Model file for the job. Use its own axes, mm. Round coordinates to 2 decimals unless told otherwise and drop trailing zeros. Write each loop counter-clockwise with the first axis right and the second up, starting at its lowest first coordinate (ties: lowest second). Pieces come first, ordered by that corner, then holes. Notation, with made-up numbers: (15.5, -5) - (23.5, -5) arc R28 ccw to (23.5, 23) - close; hole circle Ø8 at (76.5, 36). An arc over 180 degrees is marked (long way). Answer as a JSON object with one key per item and string values. Group by question number.
from build123d import *

# Parameters (mm, degrees)
SKETCH1_W           = 70
SKETCH1_H           = 200
BOSS_EXTRUDE1_DEPTH = 15
SKETCH1_3_R         = 7.5
CUT_EXTRUDE1_DEPTH  = 5
FILLET1_R           = 15


with BuildPart() as part:
    # Sketch1 → Boss-Extrude1 (new body)
    with BuildSketch(Plane(origin=(0, 0, 0), x_dir=(0, 0, -1), z_dir=(1, 0, 0))):
        Rectangle(SKETCH1_W, SKETCH1_H)
    extrude(amount=BOSS_EXTRUDE1_DEPTH)

    # Sketch1<3> → Cut-Extrude1 (cut)
    with BuildSketch(Plane(origin=(0, 0, 0), x_dir=(0, 0, -1), z_dir=(1, 0, 0))):
        with Locations((0, 80)):
            Circle(SKETCH1_3_R)
        with Locations((0, -80)):
            Circle(SKETCH1_3_R)
    extrude(amount=CUT_EXTRUDE1_DEPTH, mode=Mode.SUBTRACT)

    # Fillet1
    fillet1_edges = [part.edges().sort_by_distance(p)[0] for p in [
        (7.5, -100, -35),
        (7.5, -100, 35),
        (7.5, 100, 35),
        (7.5, 100, -35),
    ]]
    fillet(fillet1_edges, radius=FILLET1_R)


solid = part.part
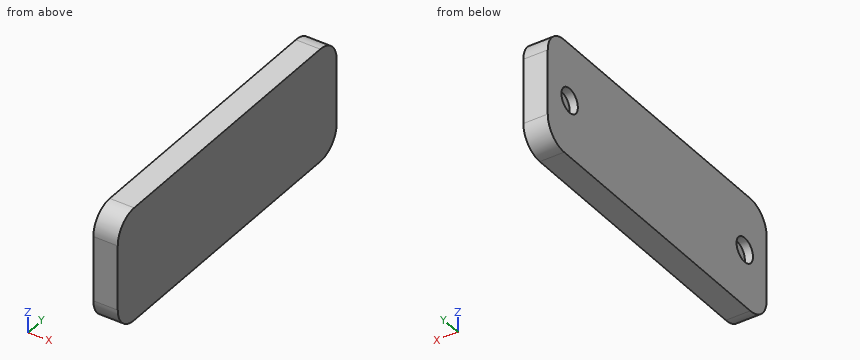
(1) Drill centre lines: line 1 (Y direction, x = 3, z = 0); line 2 (Y direction, x = 9, z = -28); line 3 (Y direction, x = 2.75, z = 26). Where is each one in solid material? Low to high. Write a range as from..to.
(2) Slice it at B-B (z = 0). Write the cut outline in (x, y).
(3) Flat gauge pin, fed straight in: pin 1 (9 mm diameter, centred on y = -80, z = 0, fed in from -X). Where does the tip first touch, or does it go through?
(4) Slice it at A-A (y = -80). Write the cut outline in (x, z), then the cut area to 3 significant figures.
Answer:
{
 "1": {"line 1": "-100..-87.5, -72.5..72.5, 87.5..100", "line 2": "-97.69..97.69", "line 3": "-98.75..98.75"},
 "2": {"outline": "(0, -100) - (15, -100) - (15, 100) - (0, 100) - (0, 87.5) - (5, 87.5) - (5, 72.5) - (0, 72.5) - (0, -72.5) - (5, -72.5) - (5, -87.5) - (0, -87.5) - close"},
 "3": {"pin 1": "x = 5"},
 "4": {"outline": "(0, -35) - (15, -35) - (15, 35) - (0, 35) - (0, 7.5) - (5, 7.5) - (5, -7.5) - (0, -7.5) - close", "area": "975 mm²"}
}
